Design review of the part built by this model. Coordinates are the model's own, in mm. Face numbers are marked on the shaded views. A direction names the side the tool comes from. Give positions to 0.01 mm unless a question says otherwise; leave off trailing zeros. Loops run counter-clockwise (first coordinate to the right, second up) from the corner with the lowest first, then second, coordinate; pieces in that order, holes last. Notation, with made-up numbers: (64, 2) -> (99, 2) arc R19 cw to (99, 34) -> close; hole circle Ø5 at (14, 30). An arc over 180 degrees is marked (long way). Use CSV: the item, a comma, the result in double quotes. Start each with the question number.
Item 1: We need section D-D (y = 9). State the section outline as (x, z) points, plus the area to 3 significant figures.
Item 2: Wall thickness on line 1 along X through (y, z) = (3.25, 0); line 2 along X through (y, z) = (6.25, 0); line 3 along Y through (x, z) = (-8.25, 11): over which ranges is each line inside the solid? List them lowest first. Write a range as from..to.
Item 3: The part is to be moulded in two halves that separate along Z. For the marked faces 3, 4 and 5, say which applies: +Z half, -Z half, draft (parallel to the pull), parting line (faces both ways), or undercut.
Item 4: We need section A-A (z = 0). State the section outline as (x, y) points, plus the area to 3 significant figures.
Item 5: For the marked faces 1 and 2, list the 3-axis set-ups (+Z, -Z, +X, -X, +Y, -Y) from which the entire face can be reached by the end or side of a thin tool; tool diameter is ignored.
Item 6: We need section C-C (x = 0). State the section outline as (y, z) points, plus the area to 3 significant figures.
Item 7: We need section B-B (y = 1.25). State the section outline as (x, z) points, plus the area to 3 significant figures.
Item 8: Clearance check with flat-ended pins moving along their axes: pin 1 (1.5 mm diameter, centred on x = 6.5, y = 6.5, fed in from -Z); pin 2 (6 mm diameter, centred on x = 0, z = -18.5, fed in from +Y); pin 3 (4 mm diameter, centred on x = -8.5, z = 6.5, fed in from -Y); pin 4 (4 mm diameter, centred on x = 8.5, z = -7, fed in from +Y). State where each tip first meets the part, or that it passes through.
from build123d import *

# Parameters (mm, degrees)
SKETCH1_R           = 2.55
BOSS_EXTRUDE1_DEPTH = 4
SKETCH2_R           = 13.25
BOSS_EXTRUDE2_DEPTH = 4.5
SKETCH3_R           = 12
CUT_EXTRUDE1_DEPTH  = 1
SKETCH4_R           = 6
BOSS_EXTRUDE3_DEPTH = 5
SKETCH5_R           = 4
CUT_EXTRUDE2_DEPTH  = 31.24070105


with BuildPart() as part:
    # Sketch1 → Boss-Extrude1 (new body)
    with BuildSketch(Plane(origin=(0, 0, 0), x_dir=(1, 0, 0), z_dir=(0, 1, 0))):
        with BuildLine():
            Line((4.959164878, 20.878378378), (12.17249561, 5.837837838))
            ThreePointArc((12.17249561, 5.837837838), (13.5, 0), (12.17249561, -5.837837838))
            Line((12.17249561, -5.837837838), (4.959164878, -20.878378378))
            ThreePointArc((4.959164878, -20.878378378), (0, -24), (-4.959164878, -20.878378378))
            Line((-4.959164878, -20.878378378), (-12.17249561, -5.837837838))
            ThreePointArc((-12.17249561, -5.837837838), (-13.5, 0), (-12.17249561, 5.837837838))
            Line((-12.17249561, 5.837837838), (-4.959164878, 20.878378378))
            ThreePointArc((-4.959164878, 20.878378378), (0, 24), (4.959164878, 20.878378378))
        make_face()
        with Locations(Location((0, 18.5, 0), (0, 0, 270))):
            Circle(SKETCH1_R, mode=Mode.SUBTRACT)
        with Locations(Location((0, -18.5, 0), (0, 0, 270))):
            Circle(SKETCH1_R, mode=Mode.SUBTRACT)
    extrude(amount=BOSS_EXTRUDE1_DEPTH)

    # Sketch2 → Boss-Extrude2 (add)
    with BuildSketch(Plane(origin=(0, 4, 0), x_dir=(1, 0, 0), z_dir=(0, 1, 0))):
        with Locations(Location((0, 0, 0), (0, 0, 270))):
            Circle(SKETCH2_R)
    extrude(amount=BOSS_EXTRUDE2_DEPTH)

    # Sketch3 → Cut-Extrude1 (cut)
    with BuildSketch(Plane(origin=(0, 8.5, 0), x_dir=(1, 0, 0), z_dir=(0, 1, 0))):
        with Locations(Location((0, 0, 0), (0, 0, 270))):
            Circle(SKETCH3_R)
    extrude(amount=-CUT_EXTRUDE1_DEPTH, mode=Mode.SUBTRACT)

    # Sketch4 → Boss-Extrude3 (add)
    with BuildSketch(Plane(origin=(0, 7.5, 0), x_dir=(1, 0, 0), z_dir=(0, 1, 0))):
        with Locations(Location((0, 0, 0), (0, 0, 270))):
            Circle(SKETCH4_R)
    extrude(amount=BOSS_EXTRUDE3_DEPTH)

    # Sketch5 → Cut-Extrude2 (cut, through all)
    with BuildSketch(Plane(origin=(0, 12.5, 0), x_dir=(1, 0, 0), z_dir=(0, 1, 0))):
        with Locations(Location((0, 0, 0), (0, 0, 270))):
            Circle(SKETCH5_R)
    extrude(amount=-CUT_EXTRUDE2_DEPTH, mode=Mode.SUBTRACT)


solid = part.part
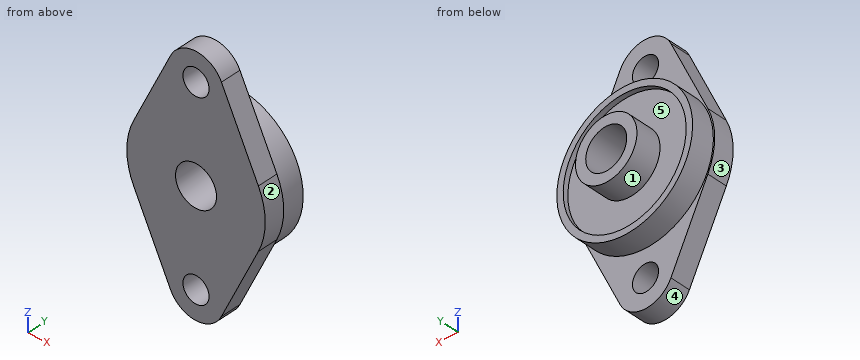
Results found:
1,outline,"circle Ø12 at (0, 0); hole circle Ø8 at (0, 0)"
1,area,"62.8 mm²"
2,line 1,"-13.5..-4, 4..13.5"
2,line 2,"-13.25..-4, 4..13.25"
2,line 3,"0..4"
3,face 3,"parting line"
3,face 4,"-Z half"
3,face 5,"undercut"
4,outline,"(-13.5, 0) -> (-4, 0) -> (-4, 12.5) -> (-6, 12.5) -> (-6, 7.5) -> (-12, 7.5) -> (-12, 8.5) -> (-13.25, 8.5) -> (-13.25, 4) -> (-13.5, 4) -> close; (4, 0) -> (13.5, 0) -> (13.5, 4) -> (13.25, 4) -> (13.25, 8.5) -> (12, 8.5) -> (12, 7.5) -> (6, 7.5) -> (6, 12.5) -> (4, 12.5) -> close"
4,area,"163 mm²"
5,face 1,"+Y"
5,face 2,"+X, +Y, -Y"
6,outline,"(0, -24) -> (4, -24) -> (4, -21.05) -> (0, -21.05) -> close; (0, -15.95) -> (4, -15.95) -> (4, -13.25) -> (8.5, -13.25) -> (8.5, -12) -> (7.5, -12) -> (7.5, -6) -> (12.5, -6) -> (12.5, -4) -> (0, -4) -> close; (0, 4) -> (12.5, 4) -> (12.5, 6) -> (7.5, 6) -> (7.5, 12) -> (8.5, 12) -> (8.5, 13.25) -> (4, 13.25) -> (4, 15.95) -> (0, 15.95) -> close; (0, 21.05) -> (4, 21.05) -> (4, 24) -> (0, 24) -> close"
6,area,"206 mm²"
7,outline,"(-12.17, -5.84) -> (-4.96, -20.88) arc R5.5 ccw to (4.96, -20.88) -> (12.17, -5.84) arc R13.5 ccw to (12.17, 5.84) -> (4.96, 20.88) arc R5.5 ccw to (-4.96, 20.88) -> (-12.17, 5.84) arc R13.5 ccw to start; hole circle Ø8 at (0, 0); hole circle Ø5.1 at (0, -18.5); hole circle Ø5.1 at (0, 18.5)"
7,area,"774 mm²"
8,pin 1,"z = -11.94"
8,pin 2,"y = 4"
8,pin 3,"y = 0"
8,pin 4,"y = 8.5"
